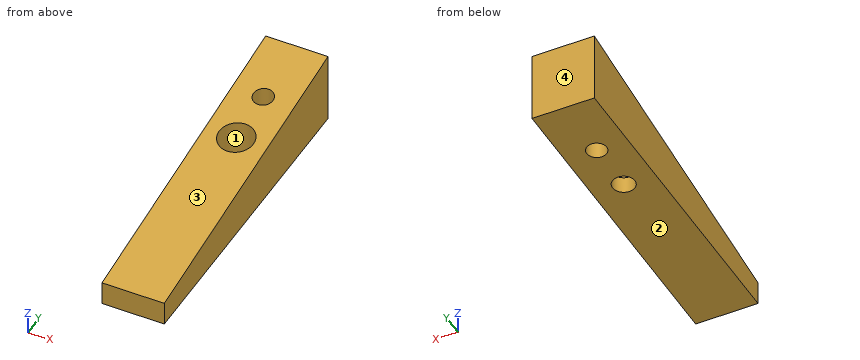
```python
from build123d import *

# Parameters (mm, degrees)
F1_DEPTH = 3.9
F3_D     = 2.5
F3_DEPTH = 12.7
F4_D     = 2.5
F4_DEPTH = 12.7


with BuildPart() as f1:
    # F0 (on Right) → F1 (new body, symmetric)
    with BuildSketch(Plane.YZ):
        Polygon((-9.4, 0), (-7, 0), (-7, 7.95), (-9.4, 7.59), align=None)
        Polygon((-40, 0), (-16.2, 0), (-16.2, 2.11), (-17, 2.11), (-17, 4.11), (-17, 6.45), (-40, 3), align=None)
        Polygon((-14.8, 0), (-13.4, 0), (-13.4, 2.11), (-12.6, 2.11), (-12.6, 4.11), (-12.6, 7.11), (-14.8, 6.78), align=None)
        Polygon((-7, 0), (0, 0), (0, 9), (-7, 7.95), align=None)
        Polygon((-16.2, 0), (-14.8, 0), (-14.8, 6.78), (-17, 6.45), (-17, 4.11), (-17, 2.11), (-16.2, 2.11), align=None)
        Polygon((-13.4, 0), (-9.4, 0), (-9.4, 7.59), (-12.6, 7.11), (-12.6, 4.11), (-12.6, 2.11), (-13.4, 2.11), align=None)
    extrude(amount=F1_DEPTH, both=True)

    # F3
    with Locations(Plane(origin=(0, 0, 0), x_dir=(1, 0, 0), z_dir=(0, 0, -1))):
        with Locations((0, 8.200222)):
            Hole(F3_D / 2, depth=F3_DEPTH)

    # F4
    with Locations(Plane(origin=(0, 0, 0), x_dir=(1, 0, 0), z_dir=(0, 0, -1))):
        with Locations((0, 14.799741)):
            Hole(F4_D / 2, depth=F4_DEPTH)

    # F0 (on Right) → F5 (revolve, cut)
    with BuildSketch(Plane.YZ):
        Polygon((-14.8, 0), (-13.4, 0), (-13.4, 2.11), (-12.6, 2.11), (-12.6, 4.11), (-12.6, 7.11), (-14.8, 6.78), align=None)
    revolve(axis=Axis((0, -14.8, 3.39), (0, 0, 1)), mode=Mode.SUBTRACT)


solid = f1.part
```
Geometry check sheet. Reference: the model listing, model coordinates, mm. Face numbers are marked on the shaded views. Round coordinates to 2 decimals unless told otherwise and drop trailing zeros. Loops run counter-clockwise (first coordinate to the right, second up) from the corner with the lowest first, then second, coordinate; pieces in that order, holes last. Notation, with made-up numbers: (42, 20.25) -> (88, 20.25) arc R22 ccw to (88, 31.25) -> close; hole circle Ø4 at (70, 3). An arc over 180 degrees is marked (long way). Use a Markdown table: item, result.
(1) Sectioned sample at B-B (x = 0). Enter the section's corners in (y, z), then the cut area to 3 significant figures.
Calculated:
| item | result |
|---|---|
| outline | (-40, 0) -> (-16.2, 0) -> (-16.2, 2.11) -> (-17, 2.11) -> (-17, 6.45) -> (-40, 3) -> close; (-13.4, 0) -> (-9.45, 0) -> (-9.45, 7.58) -> (-12.6, 7.11) -> (-12.6, 2.11) -> (-13.4, 2.11) -> close; (-6.95, 0) -> (0, 0) -> (0, 9) -> (-6.95, 7.96) -> close |
| area | 194 mm² |
(2) Sectioned sample at C-C (z = 1.25). Enter the section's corners in (x, y), then the cut area to 3 significant figures.
Calculated:
| item | result |
|---|---|
| outline | (-3.9, -40) -> (3.9, -40) -> (3.9, 0) -> (-3.9, 0) -> close; hole circle Ø2.8 at (0, -14.8); hole circle Ø2.5 at (0, -8.2) |
| area | 301 mm² |
(3) Scan lines: probe 1 along Y at (x, z) = (0, 1.2); probe 2 along X at (y, z) = (-14.8, 0.5); probe 3 along Y at (x, z) = (-0.75, 2.5). Record each from-to range of solid material in increasing order.
Calculated:
| item | result |
|---|---|
| probe 1 | -40 to -16.2, -13.4 to -9.45, -6.95 to 0 |
| probe 2 | -3.9 to -1.4, 1.4 to 3.9 |
| probe 3 | -40 to -16.87, -12.73 to -9.2, -7.2 to 0 |
(4) Mould release check, pull along Y, two halves, no side actions. Record for the marked faces 1, 2, 3 and 4: released by +Y, released by -Y, zero draft, split by the parting line, or undercut.
Calculated:
| item | result |
|---|---|
| face 1 | undercut |
| face 2 | zero draft |
| face 3 | released by -Y |
| face 4 | released by +Y |
(5) Sectioned sample at D-D (y = -31). Enter the section's corners in (x, z), then the cut area to 3 significant figures.
Calculated:
| item | result |
|---|---|
| outline | (-3.9, 0) -> (3.9, 0) -> (3.9, 4.35) -> (-3.9, 4.35) -> close |
| area | 33.9 mm² |
(6) Go/stop test with flat-tipped pins: P1, Ø4, axis at x = 2, y = -19, coming from the +Z side; P2, Ø3, axis at x = 0, y = -8.2, coming from the +Z side (3 decimals); P3, Ø1, axis at x = 1, y = -22.5, coming from the +Z side. Record where each tip stops, or that it passes through.
Calculated:
| item | result |
|---|---|
| P1 | z = 6.45 |
| P2 | z = 7.995 |
| P3 | z = 5.7 |
(7) Sectioned sample at A-A (y = -14.8). Enter the section's corners in (x, z).
Calculated:
| item | result |
|---|---|
| outline | (-3.9, 0) -> (-1.4, 0) -> (-1.4, 2.11) -> (-2.2, 2.11) -> (-2.2, 6.78) -> (-3.9, 6.78) -> close; (1.4, 0) -> (3.9, 0) -> (3.9, 6.78) -> (2.2, 6.78) -> (2.2, 2.11) -> (1.4, 2.11) -> close |
